```python
from build123d import *

# Parameters (mm, degrees)
F0_R     = 190.5
F1_DEPTH = 762
F2_W     = 203.2
F2_H     = 203.2
F3_DEPTH = 76.2
F3_TAPER = -1


with BuildPart() as f1:
    # F0 (on Top) → F1 (new body)
    with BuildSketch(Plane.XY):
        Circle(F0_R)
    extrude(amount=F1_DEPTH)

    # F2 (on face) → F3 (cut)
    with BuildSketch(Plane.XY.offset(762)):
        Rectangle(F2_W, F2_H)
    extrude(amount=-F3_DEPTH, taper=F3_TAPER, mode=Mode.SUBTRACT)

    # F4: F1 across face


with BuildPart() as f1_1:
    add(f1.part)
    add(f1.part.mirror(Plane(origin=(0, 0, 0), x_dir=(1, 0, 0), z_dir=(0, 0, -1))))


solid = f1_1.part
```
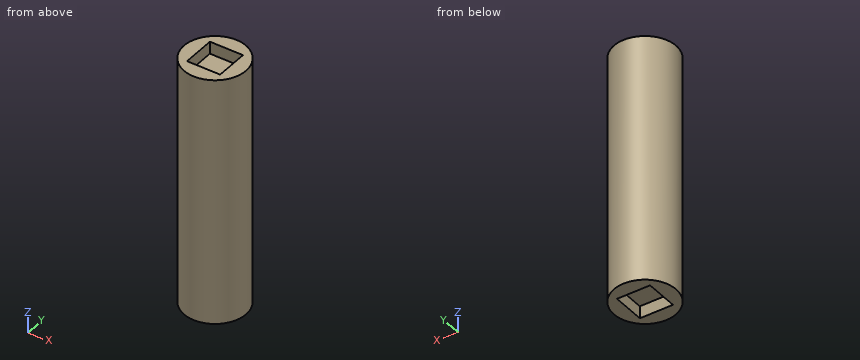
The listing builds one solid part. Answer for the finished solid, in the listing's coordinates (mm). Give positions to 0.01 mm unless a question says otherwise; leave off trailing zeros. Order: outer loops, then holes, each group sorted by start corner. A loop starts at its lowest first (then second) coordinate and runs counter-clockwise, first axis right, second up.
Item 1: The part is cut by section B-B, the plane x = 138.5. Give the vertices of the cut face in (y, z), and give its area (3 significant figures).
From the geometry:
outline: (-130.8, -762) - (130.8, -762) - (130.8, 762) - (-130.8, 762) - close
area: 399,000 mm2
Item 2: The part is cut by section C-C, the plane y = 133. Give the vertices of the cut face in (x, z), and give its area (3 significant figures).
From the geometry:
outline: (-136.39, -762) - (136.39, -762) - (136.39, 762) - (-136.39, 762) - close
area: 416,000 mm2
Item 3: The part is cut by section A-A, the plane z = 52.5. Give the vertices of the cut face in (x, y), and give its area (3 significant figures).
From the geometry:
outline: circle Ø381 at (0, 0)
area: 114,000 mm2
Item 4: Find the intervals of material crossed by probe 1 along Z at (x, y) = (7.5, -40); probe 2 along Y at (x, z) = (-160.5, 307); probe 3 along Y at (x, z) = (-42, -693), in increasing order.
From the geometry:
probe 1: z = -685.8 to 685.8
probe 2: y = -102.62 to 102.62
probe 3: y = -185.81 to -102.8, 102.8 to 185.81
Item 5: Given pin 1 Ø3 at (x, z) = (103.5, 540.5) entering from +Y; pin 2 Ø3 at (y, z) = (117, 171.5) entering from -X; pin 3 Ø5 at (x, z) = (141, -8.5) entering from -Y, each flat-ended and moving along its own axis, determine where each tip first touches the part or whether it passes through.
From the geometry:
pin 1: stops at y = 160.89
pin 2: stops at x = -151.49
pin 3: stops at y = -130.8
